Check sheet for the modelled part. Datum: model origin and axes. Units: mm. Face numbers are marked on the shaded views. A direction names the side the tool comes from. Give positions to 0.01 mm unless a question says otherwise; leave off trailing zeros. Order: outer loops, then holes, each group sorted by start corner. A loop starts at its lowest first (then second) coordinate and runs counter-clockwise, first axis right, second up.
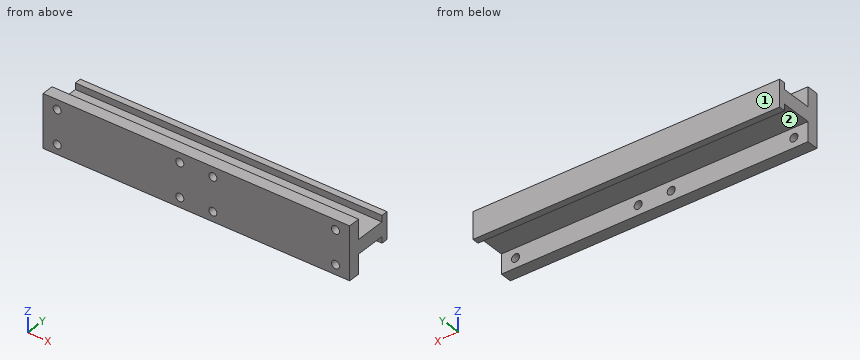
```python
from build123d import *

# Parameters (mm, degrees)
SKETCH1_W           = 130
SKETCH1_H           = 5
BOSS_EXTRUDE1_DEPTH = 22.5
SKETCH3_W           = 3
SKETCH3_H           = 3
SKETCH3_H_2         = 10
BOSS_EXTRUDE2_DEPTH = 130
CUT_EXTRUDE1_REACH  = 134.875
SKETCH4_R           = 1.7


with BuildPart() as part:
    # Sketch1 → Boss-Extrude1 (new body)
    with BuildSketch(Plane.XY):
        with Locations((65, 2.5)):
            Rectangle(SKETCH1_W, SKETCH1_H)
    extrude(amount=BOSS_EXTRUDE1_DEPTH)

    # Sketch3 → Boss-Extrude2 (add)
    with BuildSketch(Plane.ZY):
        Polygon((11.25, 18), (14.25, 18), (16.95, 18), (16.95, 20.8), (11.25, 20.8), align=None)
        Polygon((8.25, 18), (11.25, 18), (11.25, 20.8), (5.55, 20.8), (5.55, 18), align=None)
        with Locations((9.75, 16.5)):
            Rectangle(SKETCH3_W, SKETCH3_H)
        with Locations((12.75, 16.5)):
            Rectangle(SKETCH3_W, SKETCH3_H)
        with Locations((12.75, 10)):
            Rectangle(SKETCH3_W, SKETCH3_H_2)
        with Locations((9.75, 10)):
            Rectangle(SKETCH3_W, SKETCH3_H_2)
    extrude(amount=-BOSS_EXTRUDE2_DEPTH)

    # Sketch4 → Cut-Extrude1 (cut, up to next)
    with BuildSketch(Plane(origin=(0, 5, 0), x_dir=(1, 0, 0), z_dir=(0, 1, 0)), mode=Mode.PRIVATE) as cut_extrude1_sk1:
        with Locations(Location((6, -18.375, 0), (0, 0, 270))):
            Circle(SKETCH4_R)
    cut_extrude1_tool1 = extrude(cut_extrude1_sk1.sketch, amount=-CUT_EXTRUDE1_REACH, mode=Mode.PRIVATE) & part.part
    # Sketch4 → Cut-Extrude1 (cut, up to next)
    with BuildSketch(Plane(origin=(0, 5, 0), x_dir=(1, 0, 0), z_dir=(0, 1, 0)), mode=Mode.PRIVATE) as cut_extrude1_sk2:
        with Locations(Location((58, -18.375, 0), (0, 0, 270))):
            Circle(SKETCH4_R)
    cut_extrude1_tool2 = extrude(cut_extrude1_sk2.sketch, amount=-CUT_EXTRUDE1_REACH, mode=Mode.PRIVATE) & part.part
    # Sketch4 → Cut-Extrude1 (cut, up to next)
    with BuildSketch(Plane(origin=(0, 5, 0), x_dir=(1, 0, 0), z_dir=(0, 1, 0)), mode=Mode.PRIVATE) as cut_extrude1_sk3:
        with Locations(Location((72, -18.375, 0), (0, 0, 270))):
            Circle(SKETCH4_R)
    cut_extrude1_tool3 = extrude(cut_extrude1_sk3.sketch, amount=-CUT_EXTRUDE1_REACH, mode=Mode.PRIVATE) & part.part
    # Sketch4 → Cut-Extrude1 (cut, up to next)
    with BuildSketch(Plane(origin=(0, 5, 0), x_dir=(1, 0, 0), z_dir=(0, 1, 0)), mode=Mode.PRIVATE) as cut_extrude1_sk4:
        with Locations(Location((124, -18.375, 0), (0, 0, 270))):
            Circle(SKETCH4_R)
    cut_extrude1_tool4 = extrude(cut_extrude1_sk4.sketch, amount=-CUT_EXTRUDE1_REACH, mode=Mode.PRIVATE) & part.part
    # Sketch4 → Cut-Extrude1 (cut, up to next)
    with BuildSketch(Plane(origin=(0, 5, 0), x_dir=(1, 0, 0), z_dir=(0, 1, 0)), mode=Mode.PRIVATE) as cut_extrude1_sk5:
        with Locations(Location((124, -4.125, 0), (0, 0, 270))):
            Circle(SKETCH4_R)
    cut_extrude1_tool5 = extrude(cut_extrude1_sk5.sketch, amount=-CUT_EXTRUDE1_REACH, mode=Mode.PRIVATE) & part.part
    # Sketch4 → Cut-Extrude1 (cut, up to next)
    with BuildSketch(Plane(origin=(0, 5, 0), x_dir=(1, 0, 0), z_dir=(0, 1, 0)), mode=Mode.PRIVATE) as cut_extrude1_sk6:
        with Locations(Location((72, -4.125, 0), (0, 0, 270))):
            Circle(SKETCH4_R)
    cut_extrude1_tool6 = extrude(cut_extrude1_sk6.sketch, amount=-CUT_EXTRUDE1_REACH, mode=Mode.PRIVATE) & part.part
    # Sketch4 → Cut-Extrude1 (cut, up to next)
    with BuildSketch(Plane(origin=(0, 5, 0), x_dir=(1, 0, 0), z_dir=(0, 1, 0)), mode=Mode.PRIVATE) as cut_extrude1_sk7:
        with Locations(Location((58, -4.125, 0), (0, 0, 270))):
            Circle(SKETCH4_R)
    cut_extrude1_tool7 = extrude(cut_extrude1_sk7.sketch, amount=-CUT_EXTRUDE1_REACH, mode=Mode.PRIVATE) & part.part
    # Sketch4 → Cut-Extrude1 (cut, up to next)
    with BuildSketch(Plane(origin=(0, 5, 0), x_dir=(1, 0, 0), z_dir=(0, 1, 0)), mode=Mode.PRIVATE) as cut_extrude1_sk8:
        with Locations(Location((6, -4.125, 0), (0, 0, 270))):
            Circle(SKETCH4_R)
    cut_extrude1_tool8 = extrude(cut_extrude1_sk8.sketch, amount=-CUT_EXTRUDE1_REACH, mode=Mode.PRIVATE) & part.part
    add(cut_extrude1_tool1.solids().sort_by_distance((6, 5, 18.375))[0], mode=Mode.SUBTRACT)
    add(cut_extrude1_tool2.solids().sort_by_distance((58, 5, 18.375))[0], mode=Mode.SUBTRACT)
    add(cut_extrude1_tool3.solids().sort_by_distance((72, 5, 18.375))[0], mode=Mode.SUBTRACT)
    add(cut_extrude1_tool4.solids().sort_by_distance((124, 5, 18.375))[0], mode=Mode.SUBTRACT)
    add(cut_extrude1_tool5.solids().sort_by_distance((124, 5, 4.125))[0], mode=Mode.SUBTRACT)
    add(cut_extrude1_tool6.solids().sort_by_distance((72, 5, 4.125))[0], mode=Mode.SUBTRACT)
    add(cut_extrude1_tool7.solids().sort_by_distance((58, 5, 4.125))[0], mode=Mode.SUBTRACT)
    add(cut_extrude1_tool8.solids().sort_by_distance((6, 5, 4.125))[0], mode=Mode.SUBTRACT)


solid = part.part
```
(1) Material ranges on L1, parallel to Z at x = 124, y = 1.9 (3 decimals); L2, parallel to Y at x = 26, z = 16.75; L3, parallel to Y at x = 67, z = 20, recorded low to high.
Response values:
L1: z = 0 to 2.425, 5.825 to 16.675, 20.075 to 22.5
L2: y = 0 to 5, 18 to 20.8
L3: y = 0 to 5
(2) Cross-section at D-D on y = 6.5. Enter the section's corners in (x, z).
Response values:
outline: (0, 8.25) - (130, 8.25) - (130, 14.25) - (0, 14.25) - close
(3) Cross-section at A-A on x = 58. Enter the section's corners in (y, z) (3 decimals).
Response values:
outline: (0, 0) - (5, 0) - (5, 2.425) - (0, 2.425) - close; (0, 5.825) - (5, 5.825) - (5, 8.25) - (18, 8.25) - (18, 5.55) - (20.8, 5.55) - (20.8, 16.95) - (18, 16.95) - (18, 14.25) - (5, 14.25) - (5, 16.675) - (0, 16.675) - close; (0, 20.075) - (5, 20.075) - (5, 22.5) - (0, 22.5) - close
(4) Cross-section at B-B on z = 18.5. Enter the section's corners in (x, y).
Response values:
outline: (0, 0) - (4.3, 0) - (4.3, 5) - (0, 5) - close; (7.7, 0) - (56.3, 0) - (56.3, 5) - (7.7, 5) - close; (59.7, 0) - (70.3, 0) - (70.3, 5) - (59.7, 5) - close; (73.7, 0) - (122.3, 0) - (122.3, 5) - (73.7, 5) - close; (125.7, 0) - (130, 0) - (130, 5) - (125.7, 5) - close
(5) Cross-section at C-C on x = 42. Enter the section's corners in (y, z).
Response values:
outline: (0, 0) - (5, 0) - (5, 8.25) - (18, 8.25) - (18, 5.55) - (20.8, 5.55) - (20.8, 16.95) - (18, 16.95) - (18, 14.25) - (5, 14.25) - (5, 22.5) - (0, 22.5) - close
(6) Gauge pin test, flat ends, axial feed: pin 1 Ø10 at (x, y) = (80, 15.5) entering from +Z; pin 2 Ø4 at (x, y) = (79.5, 13) entering from +Z. Record the tip position at first contact, or that the pin passes through.
Response values:
pin 1: stops at z = 16.95
pin 2: stops at z = 14.25
(7) Set-up check for the marked faces 1 and 2: record each of +Z, -Z, +X, -X, +Y, -Y from which the full face is reachable in a straight line by a thin tool's end or side.
Response values:
face 1: +Z, -Z, +X, -X, +Y
face 2: -Z, +X, -X
